Build history of the part. All positions in model axes, mm. Face numbers are marked on the shaded views. Give positions to 0.01 mm unless a question says otherwise; leave off trailing zeros. Write each loop counter-clockwise with the first axis right and the second up, starting at its lowest first coordinate (ties: lowest second). Pieces come first, ordered by that corner, then holes. Notation, with made-up numbers: (-9, 43.25) - (41, 43.25) arc R23 ccw to (41, 53.25) - close; hole circle Ø1 at (36, -7). An arc over 180 degrees is marked (long way). Use one line per item in the form item = value. Start each with the question number.
from build123d import *


with BuildPart() as part:
    # Sketch1 → Revolve1 (revolve)
    with BuildSketch(Plane.XY):
        with BuildLine():
            Line((11.36894359, -6.315125633), (11.36894359, -28.655158183))
            Line((11.36894359, -28.655158183), (23.78910836, -76.005260823))
            ThreePointArc((23.78910836, -76.005260823), (23.619975063, -81.109245479), (20.312212269, -85))
            Line((20.312212269, -85), (0, -85))
            Line((0, -85), (0, -83))
            Line((0, -83), (2, -83))
            Line((2, -83), (19.724958515, -83))
            ThreePointArc((19.724958515, -83), (21.847263271, -80.130008508), (21.867118705, -76.560605981))
            Line((21.867118705, -76.560605981), (9.36894359, -28.913100051))
            Line((9.36894359, -28.913100051), (9.36894359, -4.98823705))
            ThreePointArc((9.36894359, -4.98823705), (10.882135633, -3.865208891), (10.61392266, -2))
            Line((10.61392266, -2), (11.36894359, 0))
            ThreePointArc((11.36894359, 0), (13.023652288, -3.157562817), (11.36894359, -6.315125633))
        make_face()
    revolve(axis=Axis((0, -85, 0), (0, 1, 0)))


solid = part.part
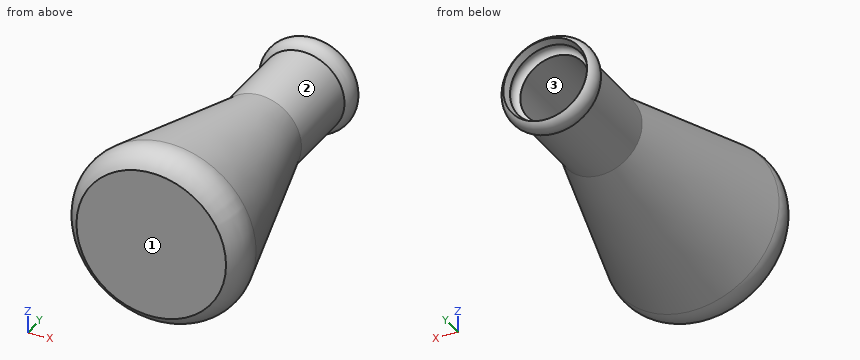
(1) Cut at D-D, the plane y = -68. Give the cut face in (x, z).
(2) Wall check: line 1 (Z direction, x = 0, y = -21); line 2 (Z direction, x = -4, y = -31). Give the ranges that are in metal, low to high. Write a range as from..to.
(3) Cut at C-C, the plane z = 0. Give the cut face in (x, y), then the cut area to 3 significant figures.
(4) Two-plate mould, pull along Z, no slides. Class the marked faces 1, 2 and 3: +Z half, -Z half, draft (parallel to the pull), parting line (faces both ways), or undercut.
(5) Cut at A-A, the plane y = -8. Give the cut face in (x, z), then the cut area to 3 significant figures.
(6) Pin check, flat tips, straight feed: pin 1 Ø4 at (x, y) = (-6, -48.5) entering from +Z; pin 2 Ø19.5 at (x, z) = (1, 7.5) entering from +Y; pin 3 Ø10 at (x, y) = (6.5, -44.5) entering from +Z; pin 4 Ø1 at (x, y) = (17.5, -55.5) entering from +Z. Stop position of each tip, or through.
(7) Cut at B-B, the plane x = 0. Give the cut face in (y, z), then the cut area to 3 significant figures.
Solution:
q1.outline = circle Ø43.38 at (0, 0); hole circle Ø39.24 at (0, 0)
q2.line_1 = -11.37..-9.37, 9.37..11.37
q2.line_2 = -11.3..-9.07, 9.07..11.3
q3.outline = (-23.79, -76.01) arc R7.75 ccw to (-20.31, -85) - (20.31, -85) arc R7.75 ccw to (23.79, -76.01) - (11.37, -28.66) - (11.37, -6.32) arc R3.84 ccw to (11.37, 0) - (10.61, -2) arc R1.84 cw to (9.37, -4.99) - (9.37, -28.91) - (21.87, -76.56) arc R5.75 cw to (19.72, -83) - (-19.72, -83) arc R5.75 cw to (-21.87, -76.56) - (-9.37, -28.91) - (-9.37, -4.99) arc R1.84 cw to (-10.61, -2) - (-11.37, 0) arc R3.84 ccw to (-11.37, -6.32) - (-11.37, -28.66) - close
q3.area = 427 mm2
q4.face_1 = draft
q4.face_2 = parting line
q4.face_3 = undercut
q5.outline = circle Ø22.74 at (0, 0); hole circle Ø18.74 at (0, 0)
q5.area = 130 mm2
q6.pin_1 = 16.31
q6.pin_2 = 0
q6.pin_3 = 16.2
q6.pin_4 = 7.11
q7.outline = (-85, -20.31) arc R7.75 ccw to (-76.01, -23.79) - (-28.66, -11.37) - (-6.32, -11.37) arc R3.84 ccw to (0, -11.37) - (-2, -10.61) arc R1.84 cw to (-4.99, -9.37) - (-28.91, -9.37) - (-76.56, -21.87) arc R5.75 cw to (-83, -19.72) - (-83, 19.72) arc R5.75 cw to (-76.56, 21.87) - (-28.91, 9.37) - (-4.99, 9.37) arc R1.84 cw to (-2, 10.61) - (0, 11.37) arc R3.84 ccw to (-6.32, 11.37) - (-28.66, 11.37) - (-76.01, 23.79) arc R7.75 ccw to (-85, 20.31) - close
q7.area = 427 mm2
